Read the model definition and answer for the solid it produces. Units are mm, in the model's axes. Give positions to 0.01 mm unless a question says otherwise; leave off trailing zeros. Write each loop counter-clockwise with the first axis right and the second up, starting at its lowest first coordinate (ties: lowest second). Pieces come first, ordered by that corner, then holes. Notation, with made-up numbers: (29, -8.5) -> (60, -8.5) arc R8 cw to (60, -3.5) -> close; hole circle Ø4 at (10, -21). An arc over 180 degrees is marked (long way). Use a Markdown table: item, result.
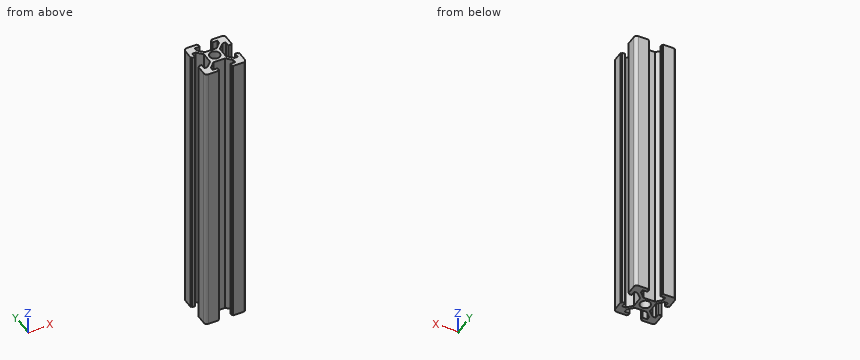
from build123d import *

# Parameters (mm, degrees)
SKETCH1_R           = 2.5
BOSS_EXTRUDE1_DEPTH = 140
SCALE_2_SCALE       = 3
SCALE_3_SCALE       = 6
SCALE_5_SCALE       = 2
SCALE_6_SCALE       = 0.25
SCALE_7_SCALE       = 0.125
SCALE_8_SCALE       = 0.25
SCALE_9_SCALE       = 4
SCALE_10_SCALE      = 4
OTHER_START         = -17.55
OTHER_1_OUTLINE_R   = 5
OTHER_1_DEPTH       = 10


# Read off the part's stored shape, not the designer's step: 孔1
with BuildPart() as part:
    # Sketch1 → Boss-Extrude1 (new body)
    with BuildSketch(Plane.XY):
        with BuildLine():
            Line((2.839339828, 3.9), (5.5, 6.560660172))
            Line((5.5, 6.560660172), (5.5, 8.2))
            Line((5.5, 8.2), (3.1, 8.2))
            Line((3.1, 8.2), (3.1, 9.5))
            Line((3.1, 9.5), (3.6, 9.5))
            Line((3.6, 9.5), (3.6, 10))
            Line((3.6, 10), (8.5, 10))
            ThreePointArc((8.5, 10), (9.560660172, 9.560660172), (10, 8.5))
            Line((10, 8.5), (10, 3.6))
            Line((10, 3.6), (9.5, 3.6))
            Line((9.5, 3.6), (9.5, 3.1))
            Line((9.5, 3.1), (8.2, 3.1))
            Line((8.2, 3.1), (8.2, 5.5))
            Line((8.2, 5.5), (6.560660172, 5.5))
            Line((6.560660172, 5.5), (3.9, 2.839339828))
            Line((3.9, 2.839339828), (3.9, -2.839339828))
            Line((3.9, -2.839339828), (6.560660172, -5.5))
            Line((6.560660172, -5.5), (8.2, -5.5))
            Line((8.2, -5.5), (8.2, -3.1))
            Line((8.2, -3.1), (9.5, -3.1))
            Line((9.5, -3.1), (9.5, -3.6))
            Line((9.5, -3.6), (10, -3.6))
            Line((10, -3.6), (10, -8.5))
            ThreePointArc((10, -8.5), (9.560660172, -9.560660172), (8.5, -10))
            Line((8.5, -10), (3.6, -10))
            Line((3.6, -10), (3.6, -9.5))
            Line((3.6, -9.5), (3.1, -9.5))
            Line((3.1, -9.5), (3.1, -8.2))
            Line((3.1, -8.2), (5.5, -8.2))
            Line((5.5, -8.2), (5.5, -6.560660172))
            Line((5.5, -6.560660172), (2.839339828, -3.9))
            Line((2.839339828, -3.9), (-2.839339828, -3.9))
            Line((-2.839339828, -3.9), (-5.5, -6.560660172))
            Line((-5.5, -6.560660172), (-5.5, -8.2))
            Line((-5.5, -8.2), (-3.1, -8.2))
            Line((-3.1, -8.2), (-3.1, -9.5))
            Line((-3.1, -9.5), (-3.6, -9.5))
            Line((-3.6, -9.5), (-3.6, -10))
            Line((-3.6, -10), (-8.5, -10))
            ThreePointArc((-8.5, -10), (-9.560660172, -9.560660172), (-10, -8.5))
            Line((-10, -8.5), (-10, -3.6))
            Line((-10, -3.6), (-9.5, -3.6))
            Line((-9.5, -3.6), (-9.5, -3.1))
            Line((-9.5, -3.1), (-8.2, -3.1))
            Line((-8.2, -3.1), (-8.2, -5.5))
            Line((-8.2, -5.5), (-6.560660172, -5.5))
            Line((-6.560660172, -5.5), (-3.9, -2.839339828))
            Line((-3.9, -2.839339828), (-3.9, 2.839339828))
            Line((-3.9, 2.839339828), (-6.560660172, 5.5))
            Line((-6.560660172, 5.5), (-8.2, 5.5))
            Line((-8.2, 5.5), (-8.2, 3.1))
            Line((-8.2, 3.1), (-9.5, 3.1))
            Line((-9.5, 3.1), (-9.5, 3.6))
            Line((-9.5, 3.6), (-10, 3.6))
            Line((-10, 3.6), (-10, 8.5))
            ThreePointArc((-10, 8.5), (-9.560660172, 9.560660172), (-8.5, 10))
            Line((-8.5, 10), (-3.6, 10))
            Line((-3.6, 10), (-3.6, 9.5))
            Line((-3.6, 9.5), (-3.1, 9.5))
            Line((-3.1, 9.5), (-3.1, 8.2))
            Line((-3.1, 8.2), (-5.5, 8.2))
            Line((-5.5, 8.2), (-5.5, 6.560660172))
            Line((-5.5, 6.560660172), (-2.839339828, 3.9))
            Line((-2.839339828, 3.9), (2.839339828, 3.9))
        make_face()
        with Locations((0, 0.235847297)):
            Circle(SKETCH1_R, mode=Mode.SUBTRACT)
    extrude(amount=BOSS_EXTRUDE1_DEPTH)


with BuildPart() as part_1:
    # 缩放比例2: scaled about (0, -0.027095247, 70)
    add(part.part.scale(SCALE_2_SCALE).moved(Location((0, 0.054190494, -140))))


with BuildPart() as part_2:
    # 缩放比例3: scaled about (0, -0.027095247, 70)
    add(part_1.part.scale(SCALE_3_SCALE).moved(Location((0, 0.135476235, -350))))


with BuildPart() as part_3:
    # 缩放比例5: scaled about (0, -0.027095249, 70)
    add(part_2.part.scale(SCALE_5_SCALE).moved(Location((0, 0.027095249, -70))))


with BuildPart() as part_4:
    # 缩放比例6: scaled about (0, -0.027095249, 70)
    add(part_3.part.scale(SCALE_6_SCALE).moved(Location((0, -0.020321437, 52.5))))


with BuildPart() as part_5:
    # 缩放比例7: scaled about (0, -0.027095249, 70)
    add(part_4.part.scale(SCALE_7_SCALE).moved(Location((0, -0.023708343, 61.25))))


with BuildPart() as part_6:
    # 缩放比例8: scaled about (0, -0.027095249, 70)
    add(part_5.part.scale(SCALE_8_SCALE).moved(Location((0, -0.020321437, 52.5))))


with BuildPart() as part_7:
    # 缩放比例9: scaled about (0, -0.027095249, 70)
    add(part_6.part.scale(SCALE_9_SCALE).moved(Location((0, 0.081285747, -210))))


with BuildPart() as part_8:
    # 缩放比例10: scaled about (0, -0.027095249, 70)
    add(part_7.part.scale(SCALE_10_SCALE).moved(Location((0, 0.081285747, -210))))

    # 孔1 outline → 孔1 (cut)
    with BuildSketch(Plane.YZ.offset(OTHER_START)):
        with Locations((7.344833538, 1.297306883)):
            Circle(OTHER_1_OUTLINE_R)
    extrude(amount=OTHER_1_DEPTH, mode=Mode.SUBTRACT)


solid = part_8.part
Item 1: Straight lines are drawn through the part: line 1 along X through (y, z) = (21, 269.5); line 2 along X through (y, z) = (-30.5, 38); line 3 along X through (y, z) = (-24.5, -130). For each, find the intervals that lie inside material, in ascending order. Write a range as [from, to].
Return value:
| item | result |
|---|---|
| line 1 | [-45, -36.9], [-25.68, -16.13], [16.13, 25.68], [36.9, 45] |
| line 2 | [-45, -24.75], [24.75, 45] |
| line 3 | [-45, -36.9], [-29.37, -19.82], [19.82, 29.37], [36.9, 45] |
Item 2: A cutting plane is placed at A-A (x = 0). Give the vertices of the cut face in (y, z), then the cut area to 3 significant figures.
Return value:
| item | result |
|---|---|
| outline | (-17.46, -245) -> (-10.09, -245) -> (-10.09, 385) -> (-17.46, 385) -> close; (12.41, -245) -> (17.64, -245) -> (17.64, 385) -> (12.41, 385) -> close |
| area | 7,940 mm^2 |
Item 3: Each of these flat-tipped pins is pushed along its axis until it touches: P1, Ø13, axis at x = -3, z = -2.5, coming from the +Y side; P2, Ø0.7, axis at y = 43.5, z = 180.5, coming from the +X side; P3, Ø1.8, axis at x = 41, z = 121, coming from the -Y side. Where does it stop, or does it pass through?
Return value:
| item | result |
|---|---|
| P1 | y = 17.64 |
| P2 | x = 42.99 |
| P3 | y = -44.65 |
